For this review, take the finished solid that the model builds, in its own axes (mm). Face numbers are marked on the shaded views. A direction names the side the tool comes from. Give positions to 0.01 mm unless a question says otherwise; leave off trailing zeros. Write each loop counter-clockwise with the first axis right and the second up, starting at its lowest first coordinate (ties: lowest second). Pieces come first, ordered by that corner, then holes. Notation, with made-up numbers: (-33.5, 46) -> (12.5, 46) arc R15 ccw to (12.5, 71) -> close; hole circle Ø9 at (-15.5, 33). An arc over 180 degrees is marked (long way). Write item = value, one per line.
```python
from build123d import *

# Parameters (mm, degrees)
EXTRUDE_1_DEPTH          = 20
CUT_EXTRUDE_1_DEPTH      = 8
FILLET_1_R               = 0.5
CUT_EXTRUDE_2_DEPTH      = 44.510647444
CUT_EXTRUDE_2_DEPTH_BACK = 44.510647444
SKETCH_5_R               = 4
FILLET_2_R               = 0.5


with BuildPart() as part:
    # 스케치1 → 보스-돌출1 (new, symmetric)
    with BuildSketch(Plane.XY):
        Polygon((0, 0), (18, 0), (18, -20.916), (0, -28.021), align=None)
    extrude(amount=EXTRUDE_1_DEPTH, both=True)

    # 스케치2 → 컷-돌출1 (cut, symmetric)
    with BuildSketch(Plane.XY):
        Polygon((0, -18.021), (18, -10.916), (18, 0), (0, 0), align=None)
    extrude(amount=CUT_EXTRUDE_1_DEPTH, both=True, mode=Mode.SUBTRACT)

    # 필렛1
    fillet_1_edges = [part.edges().sort_by_distance(p)[0] for p in [
        (0, 0, -14),
        (18, 0, -14),
        (9, 0, -8),
        (9, 0, 8),
        (0, 0, 14),
        (18, 0, 14),
    ]]
    fillet(fillet_1_edges, radius=FILLET_1_R)

    # 스케치5 → 컷-돌출2 (cut, two sides: drawn at the far end of the back side and taken through both)
    with BuildSketch(Plane.XY.offset(-8).offset(-CUT_EXTRUDE_2_DEPTH_BACK)):
        with Locations((9, -6.4685)):
            Circle(SKETCH_5_R)
    extrude(amount=CUT_EXTRUDE_2_DEPTH + CUT_EXTRUDE_2_DEPTH_BACK, mode=Mode.SUBTRACT)

    # 필렛2
    fillet_2_edges = [part.edges().sort_by_distance(p)[0] for p in [
        (5, -6.4685, -20),
        (5, -6.4685, 20),
    ]]
    fillet(fillet_2_edges, radius=FILLET_2_R)


solid = part.part
```
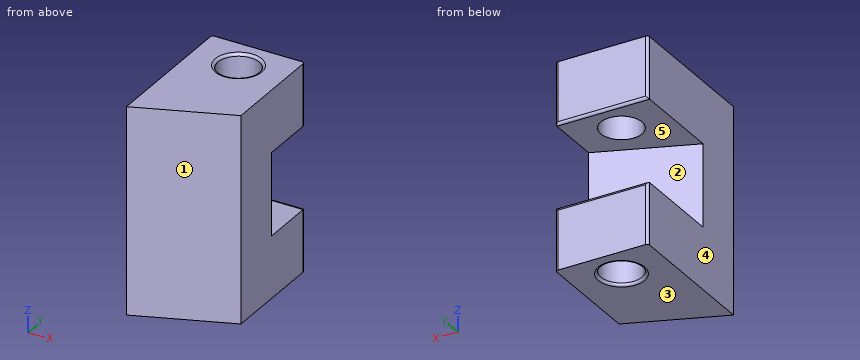
(1) Take a section at D-D (z = -5). Write out the cut boundary in (x, y).
Answers below:
outline = (0, -28.02) -> (18, -20.92) -> (18, -10.92) -> (0, -18.02) -> close
(2) For pin 1 (3 mm diameter, centred on x = 4.5, z = 6, fed in from -Y); pin 2 (1 mm diameter, centred on x = 8.5, z = -1.5, fed in from +Y); pin 3 (4 mm diameter, centred on x = 2.5, z = -11, fed in from -Y), all flat-tipped, find the tip position at first contact; note any pin that passes through.
Answers below:
pin_1 = -26.84
pin_2 = -14.47
pin_3 = -27.82
(3) Take a section at C-C (x = 16.75). Write out the cut boundary in (y, z).
Answers below:
outline = (-21.41, -20) -> (0, -20) -> (0, -8.5) arc R0.5 ccw to (-0.5, -8) -> (-11.41, -8) -> (-11.41, 8) -> (-0.5, 8) arc R0.5 ccw to (0, 8.5) -> (0, 20) -> (-21.41, 20) -> close
(4) To check wall thickness, follow probe 1 along Z at (x, y) = (17.25, -3); probe 2 along X at (y, z) = (-6.25, -15.5); probe 3 along X at (y, z) = (-9.5, 13). State the ranges of each line that lie inside material, in increasing order.
Answers below:
probe_1 = -20 to -8, 8 to 20
probe_2 = 0 to 5.01, 12.99 to 18
probe_3 = 0 to 6.39, 11.61 to 18
(5) The part is to be moulded in two halves that separate along Z. For the marked faces 1, 2 and 3, say which applies: released by +Z, released by -Z, zero draft, split by the parting line, or undercut.
Answers below:
face_1 = zero draft
face_2 = undercut
face_3 = released by -Z
(6) Take a section at A-A (z = -16.5). Write out the cut boundary in (x, y), plus the area to 3 significant figures.
Answers below:
outline = (0, -28.02) -> (18, -20.92) -> (18, -0.5) arc R0.5 ccw to (17.5, 0) -> (0.5, 0) arc R0.5 ccw to (0, -0.5) -> close; hole circle Ø8 at (9, -6.47)
area = 390 mm^2
(7) Take a section at B-B (x = 9). Write out the cut boundary in (y, z), plus the area to 3 significant figures.
Answers below:
outline = (-24.47, -20) -> (-10.97, -20) arc R0.5 ccw to (-10.47, -19.5) -> (-10.47, -8) -> (-14.47, -8) -> (-14.47, 8) -> (-10.47, 8) -> (-10.47, 19.5) arc R0.5 ccw to (-10.97, 20) -> (-24.47, 20) -> close; (-2.47, -19.5) arc R0.5 ccw to (-1.97, -20) -> (0, -20) -> (0, -8.5) arc R0.5 ccw to (-0.5, -8) -> (-2.47, -8) -> close; (-2.47, 8) -> (-0.5, 8) arc R0.5 ccw to (0, 8.5) -> (0, 20) -> (-1.97, 20) arc R0.5 ccw to (-2.47, 19.5) -> close
area = 555 mm^2
(8) Tool access review of the marked faces 4 and 5: name each direction out of +Z, -Z, +X, -X, +Y, -Y from which nothing blocks a thin tool from reaching the whole face with its end or side.
Answers below:
face_4 = +Z, -Z, -X, +Y, -Y
face_5 = -X, +Y
